Could you check a few things on this drawing? It's one solid part, dimensions in mm from its lowest x, y, z. Coordinates: 2 decimals unless noted, no trailing zeros. Order: outer loops, then holes, each group sorted by start corner. A loop starts at its lowest first (then second) coordinate and runs counter-clockwise, first axis right, second up. Notation, with made-up numbers: (-18, 20.5) -> (8, 20.5) arc R14 ccw to (8, 26.5) -> close; hole circle Ø3 at (74, 57). An arc over 180 degrees is marked (long way). Use a Markdown table: item, result. Add a question column.
1. For pin 1 Ø12 at (x, z) = (206.5, 32) entering from +Y (1 decimal); pin 2 Ø12 at (x, y) = (97.5, 7) entering from -Z; pin 3 Ø2 at (x, z) = (37, 17) entering from +Y; pin 4 Ø1.5 at (x, z) = (161.5, 66.5) entering from +Y, each with a flat end and sliding along its axis, tell me the tip position at first contact or that it passes through.
2. Suppose I cut it at B-B, the plane y = 26.5. List the corners of the cut face in (x, z) for me.
3. If I drill on line 1 along Y through (x, z) = (220, 90.5); line 2 along Y through (x, z) = (34, 90.5), over which ranges is the centre line in solid material (lowest first)? Write a range as from..to.
4. Suppose I cut it at A-A, the plane z = 63. List the corners of the cut face in (x, y) for me (1 decimal), then the cut area to 3 significant figures.
5. Suppose I cut it at C-C, the plane x = 159.5. List the corners of the cut face in (y, z) for me.
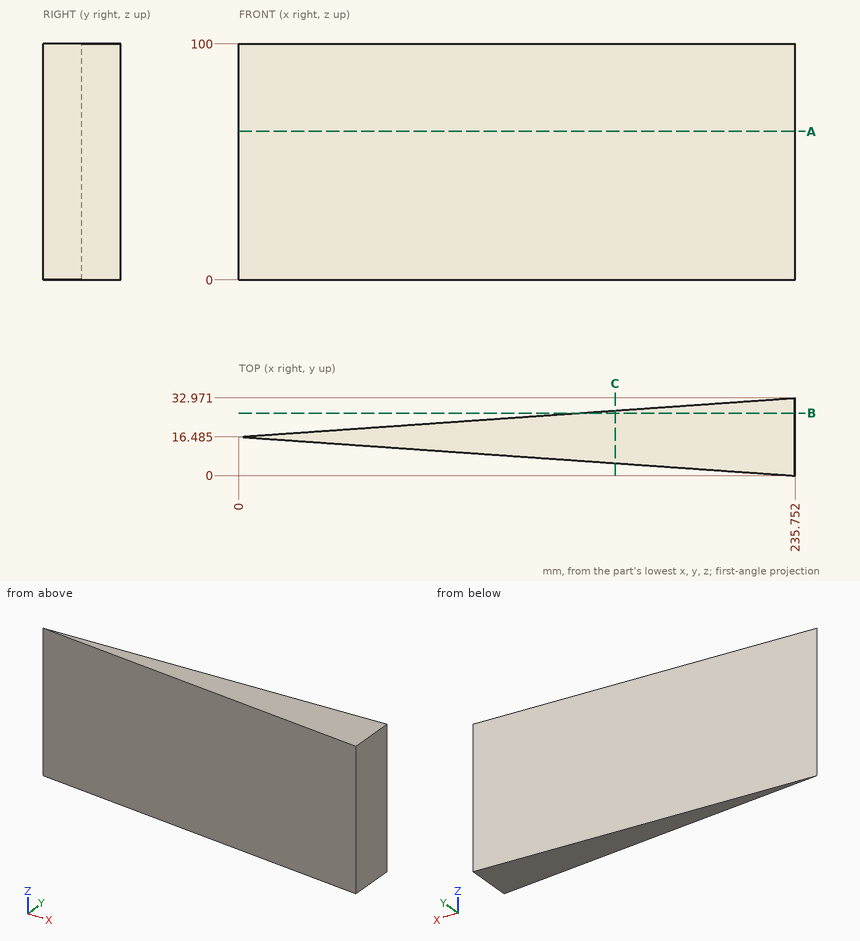
Worked out:
| question | item | result |
|---|---|---|
| 1 | pin 1 | stops at y = 31.3 |
| 1 | pin 2 | stops at z = 0 |
| 1 | pin 3 | stops at y = 19.14 |
| 1 | pin 4 | stops at y = 27.83 |
| 2 | outline | (143.22, 0) -> (235.75, 0) -> (235.75, 100) -> (143.22, 100) -> close |
| 3 | line 1 | y = 1.1..31.87 |
| 3 | line 2 | y = 14.11..18.86 |
| 4 | outline | (0, 16.5) -> (235.8, 0) -> (235.8, 33) -> close |
| 4 | area | 3,890 mm² |
| 5 | outline | (5.33, 0) -> (27.64, 0) -> (27.64, 100) -> (5.33, 100) -> close |
